```python
from build123d import *

# Parameters (mm, degrees)
SKETCH1_W           = 20
SKETCH1_H           = 9.5
BOSS_EXTRUDE1_DEPTH = 3
SKETCH2_R           = 1.75
BOSS_EXTRUDE2_DEPTH = 10.75
FILLET1_R           = 3
FILLET2_R           = 3
FILLET3_R           = 2


with BuildPart() as part:
    # Sketch1 → Boss-Extrude1 (new body)
    with BuildSketch(Plane(origin=(0, 0, 0), x_dir=(1, 0, 0), z_dir=(0, 1, 0))):
        Rectangle(SKETCH1_W, SKETCH1_H)
    extrude(amount=BOSS_EXTRUDE1_DEPTH)

    # Sketch2 → Boss-Extrude2 (add)
    with BuildSketch(Plane(origin=(0, 3, 0), x_dir=(1, 0, 0), z_dir=(0, 1, 0))):
        with BuildLine():
            Line((-14.075613498, 4.75), (-16.826627584, -3.662089657))
            ThreePointArc((-16.826627584, -3.662089657), (-14.050819142, -8.206385145), (-10, -4.75))
            Line((-10, -4.75), (-10, 4.75))
            Line((-10, 4.75), (-14.075613498, 4.75))
        make_face()
        with Locations(Location((-13.5, -4.75, 0), (0, 0, 270))):
            Circle(SKETCH2_R, mode=Mode.SUBTRACT)
    extrude(amount=-BOSS_EXTRUDE2_DEPTH)

    # Fillet1
    fillet1_edges = [part.edges().sort_by_distance(p)[0] for p in [
        (-14.075613498, -2.375, -4.75),
    ]]
    fillet(fillet1_edges, radius=FILLET1_R)

    # Fillet2
    # the kernel refuses this fillet: 3 mm, written as the material it takes off along each edge
    with BuildSketch(Plane(origin=(-10, 0, -4.75), x_dir=(-1, 0, 0), z_dir=(0, -1, 0))) as fillet2_piece_1:
        with BuildLine():
            CenterArc((3, -2.791197737), FILLET2_R, 111.502864163, 68.497135837)
            Line((0, -2.791197737), (0, 0))
            Line((0, 0), (1.900356789, 0))
        make_face()
    extrude(amount=14.727994343, mode=Mode.SUBTRACT)

    # Fillet3
    fillet3_edges = [part.edges().sort_by_distance(p)[0] for p in [
        (10, 1.5, 4.75),
        (10, 1.5, -4.75),
    ]]
    fillet(fillet3_edges, radius=FILLET3_R)


solid = part.part
```
Part model, mm, in its own coordinate system. A direction names the side the tool comes from. Coordinates: 2 decimals unless noted, no trailing zeros. Order: outer loops, then holes, each group sorted by start corner. A loop starts at its lowest first (then second) coordinate and runs counter-clockwise, first axis right, second up. Notation, with made-up numbers: (16.5, 83) -> (30.5, 83) arc R20 ccw to (30.5, 99) -> close; hole circle Ø10 at (-24, 46). An arc over 180 degrees is marked (long way). Put each result on its own line as item: value. Start each with the question number.
(1) Band-saw the part on B-B (x = -13.5). Give the cut face in (y, z).
(2) Pin check, flat tips, straight feed: pin 1 Ø3.5 at (x, y) = (-3, 2) entering from +Z; pin 2 Ø3 at (x, z) = (0.5, 0.5) entering from -Y; pin 3 Ø2 at (y, z) = (-6, 2.5) entering from +X. Stop position of each tip, or through.
(3) Band-saw the part on C-C (y = 1.25). Give the cut face in (x, z), then the cut area to 3 significant figures.
(4) Which spindle directions (+Z, -Z, +X, -X, +Y, -Y) get a long thin tool onto all of the face, cutting with end or side? Do faces 1 (the face through (-1, 1, 4.75)), 2 (the face through (-10, -4, 1)), 3 (the face through (9.4, 1.52, -4.18)). Say none if no direction does.
(5) Probe line 1 along X through (y, z) = (-3.75, 4.75); line 2 along Y through (x, z) = (4.75, -0.25); line 3 along Z through (x, y) = (5, 1). List the from-to ranges inside material, lowest first. Write a range as [from, to].
(6) Band-saw the part on A-A (z = 4.25). Give the cut face in (x, y), then the cut area to 3 significant figures.
(7) Band-saw the part on D-D (x = 6.75). Give the cut face in (y, z).
(8) Mould opens along X. For faces 4 (the face through (-2, 2, -4.75)), 5 (the face through (-10.534, -3.821, -3.668)), 6 (the face through (-15.775, -2.3, 0.445)), 7 (the face through (-11.765, -2.3, 4.522)) say: pulls with the +X half, pulls with the -X half, needs draft (parallel to the pull), parting line crosses it, or undercut.
Determined:
1. outline: (-7.75, -4.29) -> (3, -4.29) -> (3, 3) -> (-7.75, 3) -> close; (-7.75, 6.5) -> (3, 6.5) -> (3, 8.25) -> (-7.75, 8.25) -> close
2. pin 1: stops at z = 4.75
2. pin 2: stops at y = 0
2. pin 3: stops at x = -10
3. outline: (-16.83, 3.66) -> (-14.75, -2.68) arc R3 ccw to (-11.9, -4.75) -> (8, -4.75) arc R2 ccw to (10, -2.75) -> (10, 2.75) arc R2 ccw to (8, 4.75) -> (-10, 4.75) arc R3.5 ccw (long way) to start; hole circle Ø3.5 at (-13.5, 4.75)
3. area: 250 mm²
4. face 1: +Z, +X, +Y, -Y
4. face 2: +Z, -Z, +X, -Y
4. face 3: -Z, +X, +Y, -Y
5. line 1: x = [-17, -15.25], [-11.75, -10]
5. line 2: y = [0, 3]
5. line 3: z = [-4.75, 4.75]
6. outline: (-16.96, -7.75) -> (-15.18, -7.75) -> (-15.18, 3) -> (-16.96, 3) -> close; (-11.82, -7.75) -> (-10, -7.75) -> (-10, 0) -> (9.32, 0) -> (9.32, 3) -> (-11.82, 3) -> close
6. area: 96.8 mm²
7. outline: (0, -4.75) -> (3, -4.75) -> (3, 4.75) -> (0, 4.75) -> close
8. face 4: needs draft
8. face 5: pulls with the +X half
8. face 6: pulls with the -X half
8. face 7: undercut
